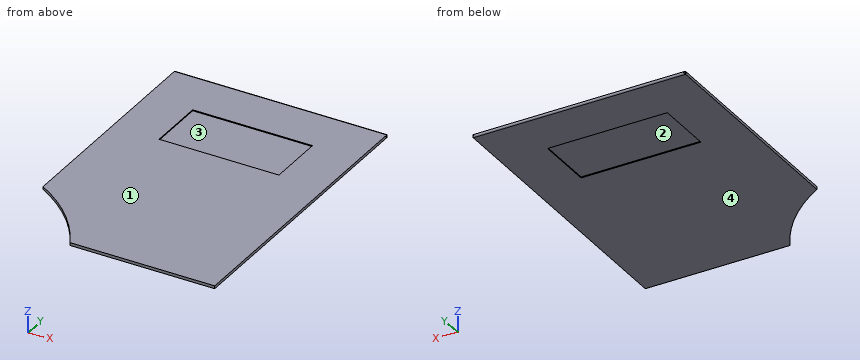
```python
from build123d import *

# Parameters (mm, degrees)
EXTRUDE_1_DEPTH     = 3
SKETCH_3_R          = 1
CUT_EXTRUDE_1_DEPTH = 435.775999416
FILLET_1_R          = 1.5
SKETCH_4_W          = 125
SKETCH_4_H          = 60
CUT_EXTRUDE_2_DEPTH = 1
CUT_EXTRUDE_3_DEPTH = 1


with BuildPart() as part:
    # 草图1 → 凸台-拉伸1 (new body)
    with BuildSketch(Plane.XY):
        with BuildLine():
            Line((-582.293881309, 65.051613642), (-431.491871246, 65.051613642))
            Line((-431.491871246, 65.051613642), (-431.491871246, 374.051613642))
            Line((-431.491871246, 374.051613642), (-653.091871246, 374.051613642))
            Line((-653.091871246, 374.051613642), (-653.091871246, 137.849062601))
            ThreePointArc((-653.091871246, 137.849062601), (-612.452891481, 106.546401187), (-582.293881309, 65.051613642))
        make_face()
    extrude(amount=EXTRUDE_1_DEPTH)

    # 草图3 → 切除-拉伸1 (cut, through all)
    with BuildSketch(Plane(origin=(-431.491871246, 0, 0), x_dir=(0, 0, -1), z_dir=(1, 0, 0))):
        with Locations((-1.5, 372.551613642)):
            Circle(SKETCH_3_R)
    extrude(amount=-CUT_EXTRUDE_1_DEPTH, mode=Mode.SUBTRACT)

    # 圆角1
    # the kernel refuses this fillet: 1.5 mm, written as the material it takes off along each edge
    with BuildSketch(Plane(origin=(-653.091871246, 374.051613642, -3.75), x_dir=(0, -1, 0), z_dir=(0, 0, 1)), Plane(origin=(-431.491871246, 374.051613642, -3.75), x_dir=(-1, 0, 0), z_dir=(0, 0, 1))) as fillet_1_piece_1:
        with BuildLine():
            CenterArc((FILLET_1_R, FILLET_1_R), FILLET_1_R, 180, 90)
            Line((0, FILLET_1_R), (0, 0))
            Line((0, 0), (FILLET_1_R, 0))
        make_face()
    extrude(amount=10.5, mode=Mode.SUBTRACT)
    with BuildSketch(Plane(origin=(-427.741871246, 374.051613642, 3), x_dir=(0, -1, 0), z_dir=(-1, 0, 0))) as fillet_1_piece_2:
        with BuildLine():
            CenterArc((FILLET_1_R, -FILLET_1_R), FILLET_1_R, 90, 90)
            Line((0, -FILLET_1_R), (0, 0))
            Line((0, 0), (FILLET_1_R, 0))
        make_face()
    extrude(amount=229.1, mode=Mode.SUBTRACT)
    with BuildSketch(Plane(origin=(-427.741871246, 374.051613642, 0), x_dir=(0, -1, 0), z_dir=(-1, 0, 0))) as fillet_1_piece_3:
        with BuildLine():
            CenterArc((FILLET_1_R, FILLET_1_R), FILLET_1_R, 180, 90)
            Line((0, FILLET_1_R), (0, 0))
            Line((0, 0), (FILLET_1_R, 0))
        make_face()
    extrude(amount=229.1, mode=Mode.SUBTRACT)

    # 草图4 → 切除-拉伸2 (cut)
    with BuildSketch(Plane(origin=(0, 0, 0), x_dir=(-1, 0, 0), z_dir=(0, 0, -1))):
        with Locations((542.291871246, 292.551613642)):
            Rectangle(SKETCH_4_W, SKETCH_4_H)
    extrude(amount=-CUT_EXTRUDE_2_DEPTH, mode=Mode.SUBTRACT)

    # 草图5 → 切除-拉伸3 (cut)
    with BuildSketch(Plane.XY.offset(3)):
        Polygon((-479.791871246, 322.551613642), (-500.741871246, 322.551613642), (-542.291871246, 292.551613642), (-500.741871246, 262.551613642), (-479.791871246, 262.551613642), align=None)
        Polygon((-500.741871246, 322.551613642), (-583.841871246, 322.551613642), (-542.291871246, 292.551613642), align=None)
        Polygon((-542.291871246, 292.551613642), (-583.841871246, 322.551613642), (-604.791871246, 322.551613642), (-604.791871246, 262.551613642), (-583.841871246, 262.551613642), align=None)
        Polygon((-542.291871246, 292.551613642), (-583.841871246, 262.551613642), (-500.741871246, 262.551613642), align=None)
    extrude(amount=-CUT_EXTRUDE_3_DEPTH, mode=Mode.SUBTRACT)


solid = part.part
```
Check sheet for the modelled part. Datum: model origin and axes. Units: mm. Face numbers are marked on the shaded views. A direction names the side the tool comes from. Round coordinates to 2 decimals unless told otherwise and drop trailing zeros. Write each loop counter-clockwise with the first axis right and the second up, starting at its lowest first coordinate (ties: lowest second). Pieces come first, ordered by that corner, then holes. Notation, with made-up numbers: (-33, 73) -> (-24, 73) arc R14 ccw to (-24, 83) -> close; hole circle Ø9 at (-3.75, 81.5). An arc over 180 degrees is marked (long way). Put each result on its own line as item: value.
(1) Sectioned sample at C-C (y = 303). Enter the section's corners in (x, z).
Values found:
outline: (-653.09, 0) -> (-604.79, 0) -> (-604.79, 1) -> (-479.79, 1) -> (-479.79, 0) -> (-431.49, 0) -> (-431.49, 3) -> (-479.79, 3) -> (-479.79, 2) -> (-604.79, 2) -> (-604.79, 3) -> (-653.09, 3) -> close
(2) Mould release check, pull along Y, two halves, no side actions. Record for the marked faces 1 and 2: released by +Y, released by -Y, zero draft, split by the parting line, or undercut.
Values found:
face 1: zero draft
face 2: undercut
(3) Tool access check on the marked faces 3 and 4. Record the directions out of +Z, -Z, +X, -X, +Y, -Y that give a thin tool (end or side, any length) a straight path to the whole face; none if there is none.
Values found:
face 3: +Z
face 4: -Z, +X, -X, +Y, -Y
(4) Sectioned sample at B-B (z = 1.5). Enter the section's corners in (x, y).
Values found:
outline: (-653.09, 137.85) arc R180 cw to (-582.29, 65.05) -> (-431.49, 65.05) -> (-431.49, 371.55) -> (-653.09, 371.55) -> close; (-652.71, 373.55) -> (-431.87, 373.55) arc R1.5 ccw to (-432.99, 374.05) -> (-651.59, 374.05) arc R1.5 ccw to start
(5) Sectioned sample at A-A (x = -576.5). Enter the section's corners in (y, z), plus the area to 3 significant figures.
Values found:
outline: (65.05, 0) -> (262.55, 0) -> (262.55, 1) -> (322.55, 1) -> (322.55, 0) -> (372.55, 0) arc R1.5 ccw to (372.55, 3) -> (322.55, 3) -> (322.55, 2) -> (262.55, 2) -> (262.55, 3) -> (65.05, 3) -> close; hole circle Ø2 at (372.55, 1.5)
area: 803 mm^2
(6) Material ranges on line 1 (Y direction, x = -518, z = 1.5); line 2 (Y direction, x = -492.5, z = 2.15); line 3 (X direction, y = 283.5, z = 2.55), recorded low to high.
Values found:
line 1: y = 65.05 to 371.55, 373.55 to 374.05
line 2: y = 65.05 to 262.55, 322.55 to 371.79, 373.31 to 373.9
line 3: x = -653.09 to -604.79, -479.79 to -431.49
(7) Go/stop test with a flat-tipped pin: pin 1 Ø6 at (x, y) = (-455.5, 122) entering from -Z. Record where the tip stops, or that it passes through.
Values found:
pin 1: stops at z = 0
